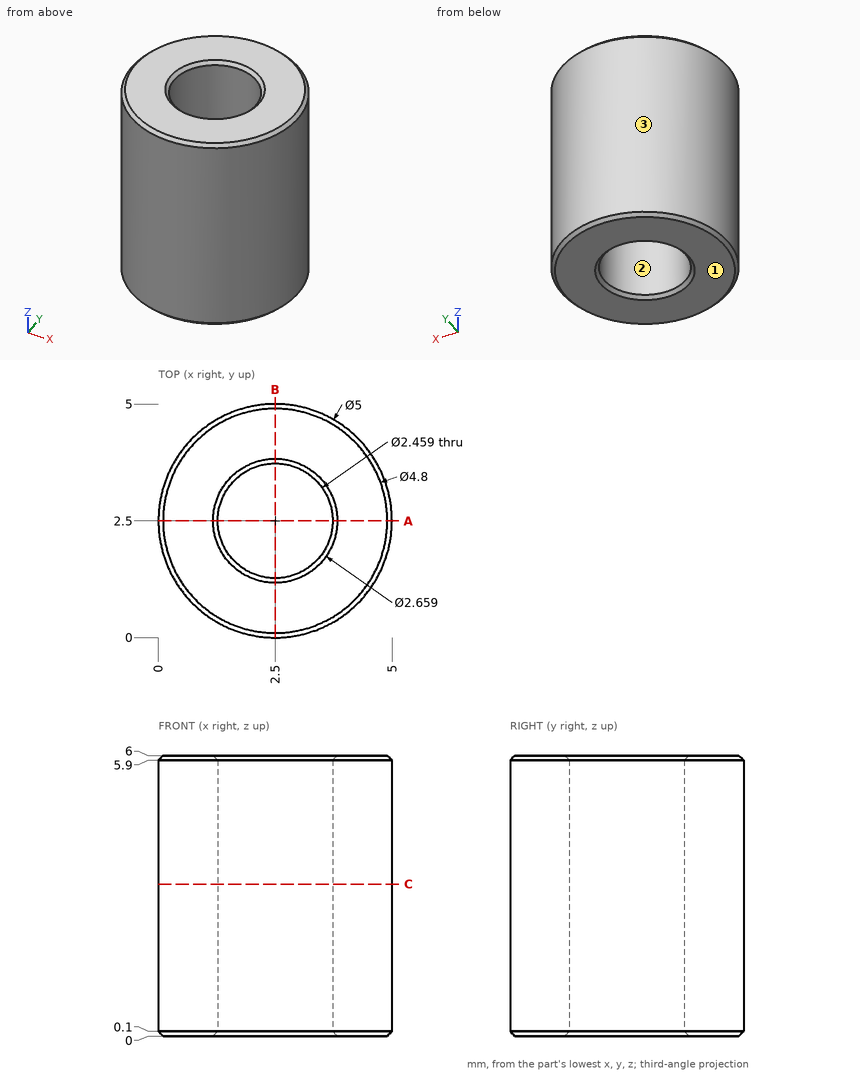
Input: dimensioned drawing with shaded views. Units: mm. Origin: part minimum x, y, z. Give positions to 0.01 mm unless a question says otherwise; leave off trailing zeros. Write each loop counter-clockwise with the first axis right and the second up, starting at its lowest first coordinate (ties: lowest second). Pieces come first, ordered by that corner, then holes.
1. Section query C-C (z = 3.25). Return the cut outline in (x, y).
2. Pull-direction query (Y, two-part tool) for the marked faces 1, 2 and 3; classes: +Y half, -Y half, draft (parallel to the pull), parting line (faces both ways), or undercut.
3. First-contact query: pin 1 (1.5 mm diameter, centred on y = 0.5, z = 2, fed in from +X); pin 2 (2 mm diameter, centred on x = 3, y = 3.5, fed in from +Z); pin 3 (1 mm diameter, centred on x = 1, z = 5.5, fed in from +Y); pin 4 (2 mm diameter, centred on x = 2.5, y = 2.5, fed in from -Z). Flat tips, straight axial feed; report the tip coordinate or a pass-through.
4. Material intervals for line 1 along Y through (x, z) = (2.5, 3.7); line 2 along X through (y, z) = (3.55, 0.65); line 3 along X through (y, z) = (1.6, 2.65), sorted ascending.
5. Section query A-A (y = 2.5). Return the cut outline in (x, z), then the cut area to 3 significant figures.
Output values:
1. outline: circle Ø5 at (2.5, 2.5); hole circle Ø2.46 at (2.5, 2.5)
2. face 1: draft
2. face 2: undercut
2. face 3: parting line
3. pin 1: stops at x = 4.67
3. pin 2: stops at z = 6
3. pin 3: stops at y = 4.79
3. pin 4: passes through
4. line 1: y = 0 to 1.27, 3.73 to 5
4. line 2: x = 0.23 to 1.86, 3.14 to 4.77
4. line 3: x = 0.17 to 1.66, 3.34 to 4.83
5. outline: (0, 0.1) - (0.1, 0) - (1.17, 0) - (1.27, 0.1) - (1.27, 5.9) - (1.17, 6) - (0.1, 6) - (0, 5.9) - close; (3.73, 0.1) - (3.83, 0) - (4.9, 0) - (5, 0.1) - (5, 5.9) - (4.9, 6) - (3.83, 6) - (3.73, 5.9) - close
5. area: 15.2 mm2
